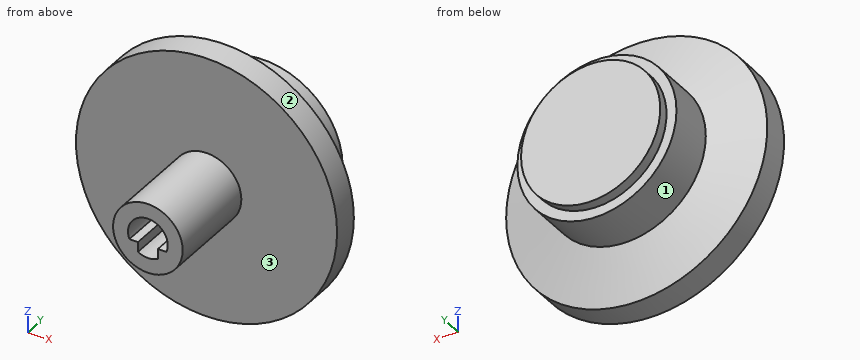
from build123d import *

# Parameters (mm, degrees)
F3_DEPTH = 20


with BuildPart() as f1:
    # F0 (on Top) → F1 (revolve)
    with BuildSketch(Plane.XY):
        Polygon((5.25, -16.505901), (5.25, -2.505901), (19.694209, -2.505901), (19.694209, 1.494099), (12, 3.994099), (12, 10.994099), (10.5, 10.994099), (10.5, 12.494099), (0, 12.494099), (0, -16.505901), align=None)
    revolve(axis=Axis((0, -14.739398, 0), (0, -1, 0)))

    # F2 (on face) → F3 (cut)
    with BuildSketch(Plane.XZ.offset(16.505901)):
        with BuildLine():
            Line((-1.5, -1.098076), (-1.5, -2.598076))
            ThreePointArc((-1.5, -2.598076), (0, -3), (1.5, -2.598076))
            Line((1.5, -2.598076), (1.5, -1.098076))
            Line((1.5, -1.098076), (2.791815, -1.098076))
            ThreePointArc((2.791815, -1.098076), (0, 3), (-2.791815, -1.098076))
            Line((-2.791815, -1.098076), (-1.5, -1.098076))
        make_face()
    extrude(amount=-F3_DEPTH, mode=Mode.SUBTRACT)


solid = f1.part
Could you check a few things on this model? Use its own coordinates, in mm. Face numbers are marked on the shaded views. A direction names the side the tool comes from. Give positions to 0.01 mm unless a question says otherwise; leave off trailing zeros. Order: outer loops, then holes, each group sorted by start corner. A loop starts at its lowest first (then second) coordinate and runs counter-clockwise, first axis right, second up. Notation, with made-up numbers: (-8, -22.75) -> (9, -22.75) arc R12 cw to (9, -15.75) -> close; hole circle Ø6 at (51.5, 76). An arc over 180 degrees is marked (long way). Return JSON: item names as keys, results as strings.
1. I need wall thicknesses on line 1 (Z direction, x = 0, y = -3.5); line 2 (Y direction, x = -8.5, z = -3.5); line 3 (Z direction, x = 0, y = -1.5). Which ranges of each line are inside material? Lowest first, please. Write a range as from..to.
Answer list:
{"line 1": "z = -5.25..-3, 3..5.25", "line 2": "y = -2.51..12.49", "line 3": "z = -19.69..-3, 3..19.69"}
2. Imagine slicing it at A-A on x = 0. List the corners of the cut face in (y, z) for me.
Answer list:
{"outline": "(-16.51, -5.25) -> (-2.51, -5.25) -> (-2.51, -19.69) -> (1.49, -19.69) -> (3.99, -12) -> (10.99, -12) -> (10.99, -10.5) -> (12.49, -10.5) -> (12.49, 10.5) -> (10.99, 10.5) -> (10.99, 12) -> (3.99, 12) -> (1.49, 19.69) -> (-2.51, 19.69) -> (-2.51, 5.25) -> (-16.51, 5.25) -> (-16.51, 3) -> (3.49, 3) -> (3.49, -3) -> (-16.51, -3) -> close"}
3. For pin 1 Ø3 at (x, z) = (10, 12) entering from -Y; pin 2 Ø1.6 at (y, z) = (-3, -2) entering from -X; pin 3 Ø12 at (y, z) = (2.5, 9.5) entering from -X, each with a flat end and sliding along its axis, tell me the tip position at first contact or that it passes through.
Answer list:
{"pin 1": "stops at y = -2.51", "pin 2": "stops at x = -19.65", "pin 3": "stops at x = -19.37"}
4. On a 3-axis mill with a long thin cutter (end or side, diameter ignored), from which of +Z, -Z, +X, -X, +Y, -Y can I reach the whole of each face in a straight line? I mean the marked faces 1, 2 and 3. Say none if no direction works.
Answer list:
{"face 1": "+Y", "face 2": "+Y, -Y", "face 3": "-Y"}
5. Imagine slicing it at B-B on y = -8.75. List the corners of the cut face in (x, z) for me, then the cut area to 3 significant figures.
Answer list:
{"outline": "circle Ø10.5 at (0, 0); hole (-2.79, -1.1) -> (-1.5, -1.1) -> (-1.5, -2.6) arc R3 ccw to (1.5, -2.6) -> (1.5, -1.1) -> (2.79, -1.1) arc R3 ccw (long way) to start", "area": "60.7 mm2"}
6. Imagine slicing it at C-C on z = 0. List the corners of the cut face in (x, y) for me, then the cut area to 3 significant figures.
Answer list:
{"outline": "(-19.69, -2.51) -> (-5.25, -2.51) -> (-5.25, -16.51) -> (-3, -16.51) -> (-3, 3.49) -> (3, 3.49) -> (3, -16.51) -> (5.25, -16.51) -> (5.25, -2.51) -> (19.69, -2.51) -> (19.69, 1.49) -> (12, 3.99) -> (12, 10.99) -> (10.5, 10.99) -> (10.5, 12.49) -> (-10.5, 12.49) -> (-10.5, 10.99) -> (-12, 10.99) -> (-12, 3.99) -> (-19.69, 1.49) -> close", "area": "463 mm2"}
